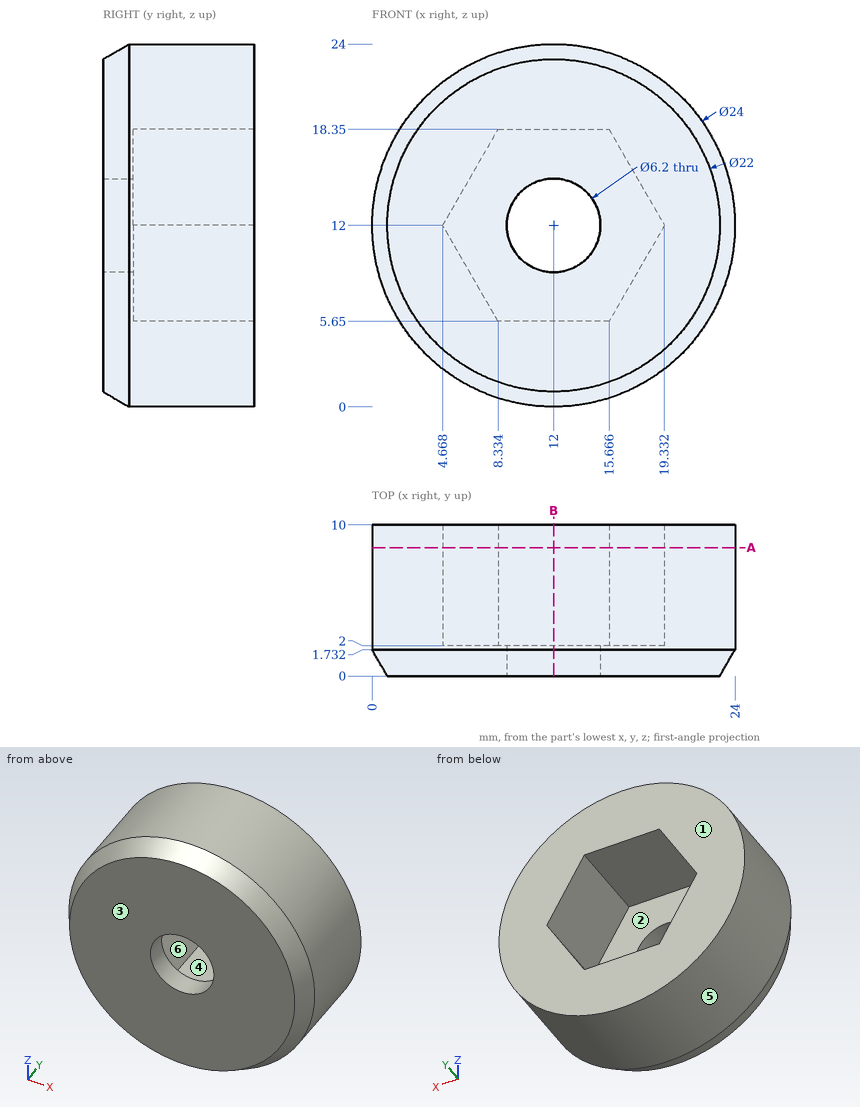
Geometry: see drawing. Coordinates: mm, zero at the bounding-box minimum. A direction names the side the tool comes from. Coordinates: 2 decimals unless noted, no trailing zeros. Order: outer loops, then holes, each group sorted by start corner. A loop starts at its lowest first (then second) coordinate and runs counter-clockwise, first axis right, second up. Notation, with made-up numbers: M 67,55.5 L 111,55.5 A13 cw 111,72.5 Z; hole C 79.5,46.5 d7. An arc over 180 degrees is marked long. Write item = value, one per line. Start each with the question number.
(1) Section B-B on x = 12. Output: boundary loops of the cut face in (y, z), and give its area (3 significant figures).
(2) Line query: line 1 along X through (y, z) = (7.75, 14.5); line 2 along Y through (x, z) = (7.75, 10.5); line 3 along X through (y, z) = (7.25, 8) (1 decimal). Output: solid intervals per line, ascending. Write a range as [from, to].
(3) Pull-direction query (Z, two-part tool) for the marked faces 3, 4, 5 and 6; classes: released by +Z, released by -Z, zero draft, split by the parting line, or undercut.
(4) Reachability of the marked faces 1 and 2 from +Z, -Z, +X, -X, +Y, -Y: full face, straight path, thin tool, end or side. Return the list, or none.
(5) First-contact query: P1, Ø2, axis at x = 8.5, y = 4, coming from the +Z side; P2, Ø4, axis at x = 21, y = 8, coming from the +Z side; P3, Ø1.5, axis at x = 13, z = 15, coming from the +Y side. Flat tips, straight axial feed; report the tip coordinate or a pass-through.
(6) Section A-A on y = 8.5. Output: boundary loops of the cut face in (x, z), and give its area (3 significant figures).
Result set:
q1.outline = M 0,1 L 1.73,0 L 10,0 L 10,5.65 L 2,5.65 L 2,8.9 L 0,8.9 Z; M 0,15.1 L 2,15.1 L 2,18.35 L 10,18.35 L 10,24 L 1.73,24 L 0,23 Z
q1.area = 124 mm²
q2.line_1 = [0.26, 6.11], [17.89, 23.74]
q2.line_2 = [0, 2]
q2.line_3 = [0.7, 7], [17, 23.3]
q3.face_3 = zero draft
q3.face_4 = undercut
q3.face_5 = split by the parting line
q3.face_6 = undercut
q4.face_1 = +Z, -Z, +X, -X, +Y
q4.face_2 = +Y
q5.P1 = 23.74
q5.P2 = 21.75
q5.P3 = 2
q6.outline = C 12,12 d24; hole M 4.67,12 L 8.33,5.65 L 15.67,5.65 L 19.33,12 L 15.67,18.35 L 8.33,18.35 Z
q6.area = 313 mm²
